Build history of the part. All positions in model axes, mm. Face numbers are marked on the shaded views. A direction names the side the tool comes from. Round coordinates to 2 decimals unless told otherwise and drop trailing zeros. Loops run counter-clockwise (first coordinate to the right, second up) from the corner with the lowest first, then second, coordinate; pieces in that order, holes last. Notation, with made-up numbers: M 46.5,47.5 L 98.5,47.5 A13 cw 98.5,69.5 Z; hole C 87,52.5 d4. An arc over 180 degrees is marked long. One line per item, written item: value.
```python
from build123d import *

# Parameters (mm, degrees)
SKETCH1_W           = 42
SKETCH1_H           = 24
BOSS_EXTRUDE1_DEPTH = 1.1176
SKETCH2_R           = 1.3
CUT_EXTRUDE1_DEPTH  = 25.21257999
SKETCH3_W           = 30
SKETCH3_H           = 14
BOSS_EXTRUDE2_DEPTH = 7.3
SKETCH4_R           = 0.5
CUT_EXTRUDE2_DEPTH  = 26.609685468
SKETCH5_W           = 9
SKETCH5_H           = 12.25
BOSS_EXTRUDE3_DEPTH = 2.5
SKETCH6_W           = 3.16
SKETCH6_H           = 1.2
BOSS_EXTRUDE4_DEPTH = 1.2


with BuildPart() as part:
    # Sketch1 → Boss-Extrude1 (new body)
    with BuildSketch(Plane.XY):
        Rectangle(SKETCH1_W, SKETCH1_H)
    extrude(amount=BOSS_EXTRUDE1_DEPTH)

    # Sketch2 → Cut-Extrude1 (cut, through all)
    with BuildSketch(Plane.XY):
        with Locations((-18.9175, 9.8975)):
            Circle(SKETCH2_R)
        with Locations((-18.9175, -9.8975)):
            Circle(SKETCH2_R)
        with Locations((18.9175, -9.8975)):
            Circle(SKETCH2_R)
        with Locations((18.9175, 9.8975)):
            Circle(SKETCH2_R)
    extrude(amount=CUT_EXTRUDE1_DEPTH, mode=Mode.SUBTRACT)

    # Sketch3 → Boss-Extrude2 (add)
    with BuildSketch(Plane.XY.offset(1.1176)):
        with Locations((1.12, 0.4)):
            Rectangle(SKETCH3_W, SKETCH3_H)
    extrude(amount=BOSS_EXTRUDE2_DEPTH)

    # Sketch4 → Cut-Extrude2 (cut, through all)
    with BuildSketch(Plane.XY):
        with Locations((18.46, 3.81)):
            Circle(SKETCH4_R)
        with Locations((18.46, 1.27)):
            Circle(SKETCH4_R)
        with Locations((18.46, -1.27)):
            Circle(SKETCH4_R)
        with Locations((18.46, -3.81)):
            Circle(SKETCH4_R)
    extrude(amount=CUT_EXTRUDE2_DEPTH, mode=Mode.SUBTRACT)

    # Sketch5 → Boss-Extrude3 (add)
    with BuildSketch(Plane(origin=(0, 0, 0), x_dir=(-1, 0, 0), z_dir=(0, 0, -1))):
        with Locations((13.14, -0.225)):
            Rectangle(SKETCH5_W, SKETCH5_H)
    extrude(amount=BOSS_EXTRUDE3_DEPTH)

    # Sketch6 → Boss-Extrude4 (add)
    with BuildSketch(Plane(origin=(0, 0, 0), x_dir=(-1, 0, 0), z_dir=(0, 0, -1))):
        with Locations((15.42, 8.8092)):
            Rectangle(SKETCH6_W, SKETCH6_H)
    extrude(amount=BOSS_EXTRUDE4_DEPTH)


solid = part.part
```
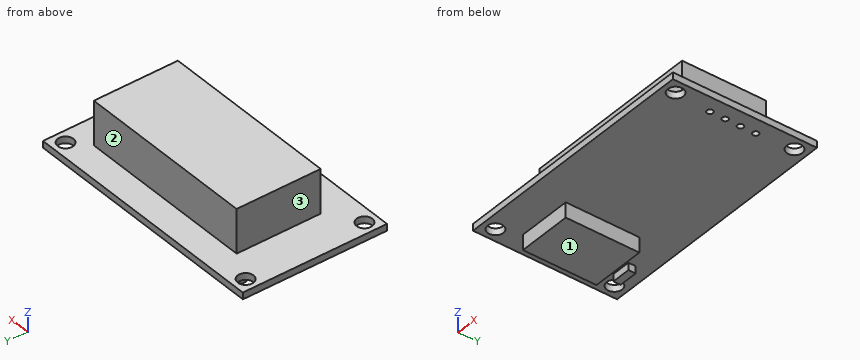
Item 1: Drop flat-ended pins along their axis: P1, Ø0.6, axis at y = 8.5, z = -0.5, coming from the -X side; P2, Ø2, axis at y = 3, z = 5, coming from the +X side; P3, Ø1, axis at x = 3.5, z = 5, coming from the -Y side. Give the stop position or say it passes through.
Check values:
P1: stops at x = -17
P2: stops at x = 16.12
P3: stops at y = -6.6
Item 2: Slice it at A-A, the plane y = -1.27. Give the cut face in (x, z), and give its area (3 significant figures).
Check values:
outline: M -21,0 L -17.64,0 L -17.64,-2.5 L -8.64,-2.5 L -8.64,0 L 17.96,0 L 17.96,1.12 L 16.12,1.12 L 16.12,8.42 L -13.88,8.42 L -13.88,1.12 L -21,1.12 Z; M 18.96,0 L 21,0 L 21,1.12 L 18.96,1.12 Z
area: 287 mm2
Item 3: Wall check: line 1 along X through (y, z) = (-1.27, 0.5); line 2 along Y through (x, z) = (-7, 4.5); line 3 along Z through (x, y) = (1, 10.5). Give the ranges that are in metal, low to high.
Check values:
line 1: x = -21 to 17.96, 18.96 to 21
line 2: y = -6.6 to 7.4
line 3: z = 0 to 1.12
Item 4: Which spindle directions (+Z, -Z, +X, -X, +Y, -Y) get a long thin tool onto all of the face, cutting with end or side? Do the marked faces 1, 2 and 3. Say none if no direction does.
Check values:
face 1: -Z, +X, -X, +Y, -Y
face 2: +Z, +X, -X, +Y
face 3: +Z, -X, +Y, -Y
Item 5: Slice it at C-C, the plane x = 18.46. Give the cut face in (y, z).
Check values:
outline: M -12,0 L -11.11,0 L -11.11,1.12 L -12,1.12 Z; M -8.68,0 L -4.31,0 L -4.31,1.12 L -8.68,1.12 Z; M -3.31,0 L -1.77,0 L -1.77,1.12 L -3.31,1.12 Z; M -0.77,0 L 0.77,0 L 0.77,1.12 L -0.77,1.12 Z; M 1.77,0 L 3.31,0 L 3.31,1.12 L 1.77,1.12 Z; M 4.31,0 L 8.68,0 L 8.68,1.12 L 4.31,1.12 Z; M 11.11,0 L 12,0 L 12,1.12 L 11.11,1.12 Z
Item 6: Slice it at B-B, the plane x = -11.5. Give the cut face in (y, z).
Check values:
outline: M -12,0 L -6.35,0 L -6.35,-2.5 L 5.9,-2.5 L 5.9,0 L 12,0 L 12,1.12 L 7.4,1.12 L 7.4,8.42 L -6.6,8.42 L -6.6,1.12 L -12,1.12 Z
Item 7: Slice it at D-D, the plane z = 7.75. Give the cut face in (x, y), and give its area (3 significant figures).
Check values:
outline: M -13.88,-6.6 L 16.12,-6.6 L 16.12,7.4 L -13.88,7.4 Z
area: 420 mm2
